Geometry: final body of the model. Coordinates: model frame, mm. A direction names the side the tool comes from. Round coordinates to 2 decimals unless told otherwise and drop trailing zeros. Write each loop counter-clockwise with the first axis right and the second up, starting at its lowest first coordinate (ties: lowest second). Pieces come first, ordered by that corner, then holes. Notation, with made-up numbers: (82.25, 29) - (124.25, 29) arc R9 cw to (124.25, 46) - close; hole circle Ø8 at (-22, 84.5). An arc over 180 degrees is marked (long way). Use a Markdown table: item, result. Add a question column.
```python
from build123d import *

# Parameters (mm, degrees)
F1_DEPTH = 1
F3_DEPTH = 1.5
F4_R     = 4
F4_R_2   = 3.5
F5_DEPTH = 2.5


with BuildPart() as f1:
    # F0 (on Front) → F1 (new body)
    with BuildSketch(Plane.XZ):
        with BuildLine():
            ThreePointArc((0, 2), (0.5857864376, 0.5857864376), (2, 0))
            Line((2, 0), (40, 0))
            ThreePointArc((40, 0), (41.4142135624, 0.5857864376), (42, 2))
            Line((42, 2), (42, 25))
            Line((42, 25), (0, 25))
            Line((0, 25), (0, 2))
        make_face()
    extrude(amount=F1_DEPTH)

    # F2 (on face) → F3 (join)
    with BuildSketch(Plane.XZ.offset(1)):
        with BuildLine():
            Line((39.75, 25), (2.25, 25))
            Line((2.25, 25), (2.25, 2))
            ThreePointArc((2.25, 2), (2.8357864376, 0.5857864376), (4.25, 0))
            Line((4.25, 0), (37.75, 0))
            ThreePointArc((37.75, 0), (39.1642135624, 0.5857864376), (39.75, 2))
            Line((39.75, 2), (39.75, 25))
        make_face()
    extrude(amount=F3_DEPTH)

    # F4 (on face) → F5 (cut, through all)
    with BuildSketch(Plane.XZ.offset(2.5)):
        with Locations((33.25, 10)):
            Circle(F4_R)
        with Locations((9.25, 6.5)):
            Circle(F4_R_2)
    extrude(amount=-F5_DEPTH, mode=Mode.SUBTRACT)


solid = f1.part
```
1) Draft query along X for faces 5 (the cylindrical face through (29.254, -1.268, 10.176)), 6 (the flat face through (21, -2.5, 13)), 7 (the cylindrical face through (5.753, -1.268, 6.654)), 8 (the cylindrical face through (41.4, -0.49, 0.57)). Return one class per face: released by +X, released by -X, zero draft, split by the parting line, or undercut.
2) Section C-C, the plane z = 6.5. Return the cut outline in (x, y), then the cut area to 3 significant figures.
3) Set-up query: faces 1 (the flat face through (39.75, -2, 13)), 2 (the cylindrical face through (39.15, -1.74, 0.57)), 3 (the cylindrical face through (2.82, -1.74, 0.6)), 4 (the flat face through (2.25, -2, 14)). Return all of +Z, -Z, +X, -X, +Y, -Y with unobstructed straight access to the full face (end or side cutting, diameter ignored); none if empty.
4) Section B-B, the plane y = -1.9. Return the cut outline in (x, z).
5) Section D-D, the plane z = 10.5. Return the cut outline in (x, y), then the cut area to 3 significant figures.
6) Material intervals for L1, parallel to Z at x = 33.5, y = -2; L2, parallel to X at y = -2.05, z = 22.25; L3, parallel to X at y = -0.95, z = 9, sorted ascending. Write a range as from..to.
7) Section A-A, the plane x = 9.25. Return the cut outline in (y, z), then the cut area to 3 significant figures.
8) Pin query (flat end, axial travel): P1, Ø6.5, axis at x = 33.25, z = 10, coming from the +Y side; P2, Ø1, axis at y = -2, z = 9, coming from the -X side; P3, Ø1.3, axis at x = 41, z = 13.5, coming from the -Y side. Return the tip coordinate at first contact, or that it passes through.
Output values:
| question | item | result |
|---|---|---|
| 1 | face 5 | undercut |
| 1 | face 6 | zero draft |
| 1 | face 7 | undercut |
| 1 | face 8 | released by +X |
| 2 | outline | (0, -1) - (2.25, -1) - (2.25, -2.5) - (5.75, -2.5) - (5.75, 0) - (0, 0) - close; (12.75, -2.5) - (31.31, -2.5) - (31.31, 0) - (12.75, 0) - close; (35.19, -2.5) - (39.75, -2.5) - (39.75, -1) - (42, -1) - (42, 0) - (35.19, 0) - close |
| 2 | area | 71.1 mm^2 |
| 3 | face 1 | +Z, -Z, +X, -Y |
| 3 | face 2 | -Z, +X, -Y |
| 3 | face 3 | -Z, -X, -Y |
| 3 | face 4 | +Z, -Z, -X, -Y |
| 4 | outline | (2.25, 2) arc R2 ccw to (4.25, 0) - (37.75, 0) arc R2 ccw to (39.75, 2) - (39.75, 25) - (2.25, 25) - close; hole circle Ø7 at (9.25, 6.5); hole circle Ø8 at (33.25, 10) |
| 5 | outline | (0, -1) - (2.25, -1) - (2.25, -2.5) - (29.28, -2.5) - (29.28, 0) - (0, 0) - close; (37.22, -2.5) - (39.75, -2.5) - (39.75, -1) - (42, -1) - (42, 0) - (37.22, 0) - close |
| 5 | area | 78.4 mm^2 |
| 6 | L1 | z = 0..6.01, 13.99..25 |
| 6 | L2 | x = 2.25..39.75 |
| 6 | L3 | x = 0..6.8, 11.7..29.38, 37.12..42 |
| 7 | outline | (-2.5, 0) - (0, 0) - (0, 3) - (-2.5, 3) - close; (-2.5, 10) - (0, 10) - (0, 25) - (-2.5, 25) - close |
| 7 | area | 45.0 mm^2 |
| 8 | P1 | passes through |
| 8 | P2 | stops at x = 2.25 |
| 8 | P3 | stops at y = -1 |
